The model under review builds one solid part; all positions refer to its coordinate system, in mm. Face numbers are marked on the shaded views. A direction names the side the tool comes from. Give positions to 0.01 mm unless a question says otherwise; leave off trailing zeros. Loops run counter-clockwise (first coordinate to the right, second up) from the corner with the lowest first, then second, coordinate; pieces in that order, holes last. Notation, with made-up numbers: (-28.5, 14) - (-3.5, 14) arc R20 cw to (-3.5, 26) - close; hole circle Ø4 at (57, 71). An arc over 180 degrees is marked (long way). Answer as a JSON object with one key per item and string values.
from build123d import *

# Parameters (mm, degrees)
F0_W     = 110
F0_H     = 30
F1_DEPTH = 10
F2_R     = 2
F3_DEPTH = 25
F4_W     = 10
F4_H     = 30
F5_DEPTH = 30
F6_R     = 2
F7_DEPTH = 25
F8_R     = 4.99999


# Not quite as in the source:
# - a fillet or chamfer is up to 0.001 mm smaller than in the source, because OpenCascade refuses the exact size
# - a feature names something its author has since deleted; it is built from what else it names


with BuildPart() as f1:
    # F0 (on Top) → F1 (new body)
    with BuildSketch(Plane.XY):
        with Locations((-55, 15)):
            Rectangle(F0_W, F0_H)
    extrude(amount=F1_DEPTH)

    # F2 (on face) → F3 (cut)
    with BuildSketch(Plane(origin=(0, 0, 0), x_dir=(1, 0, 0), z_dir=(0, 0, -1))):
        with Locations((-8, -8)):
            Circle(F2_R)
        with Locations((-73, -8)):
            Circle(F2_R)
        with BuildLine():
            Line((0, -30), (0, -15))
            Line((0, -15), (-65, -15))
            ThreePointArc((-65, -15), (-75.6066017178, -19.3933982822), (-80, -30))
            Line((-80, -30), (0, -30))
        make_face()
    extrude(amount=-F3_DEPTH, mode=Mode.SUBTRACT)

    # F4 (on face) → F5 (join)
    with BuildSketch(Plane.XY.offset(10)):
        with Locations((-105, 15)):
            Rectangle(F4_W, F4_H)
    extrude(amount=F5_DEPTH)

    # F6 (on face) → F7 (cut)
    with BuildSketch(Plane.YZ.offset(-100)):
        with Locations((7, 17)):
            Circle(F6_R)
        with Locations((7, 25)):
            Circle(F6_R)
        with Locations((15, 33)):
            Circle(F6_R)
        with Locations((7, 33)):
            Circle(F6_R)
        with Locations((15, 25)):
            Circle(F6_R)
        with Locations((15, 17)):
            Circle(F6_R)
        with Locations((23, 17)):
            Circle(F6_R)
        with Locations((23, 25)):
            Circle(F6_R)
        with Locations((23, 33)):
            Circle(F6_R)
    extrude(amount=-F7_DEPTH, mode=Mode.SUBTRACT)

    # F8 (radius 5 in the source; OpenCascade refuses exactly that, so slightly less here)
    f8_edges = [f1.edges().sort_by_distance(p)[0] for p in [
        (0, 15, 5),
        (0, 0, 5),
        (-80, 30, 5),
        (-105, 30, 40),
        (-105, 0, 40),
        (-100, 15, 10),
    ]]
    fillet(f8_edges, radius=F8_R)


solid = f1.part
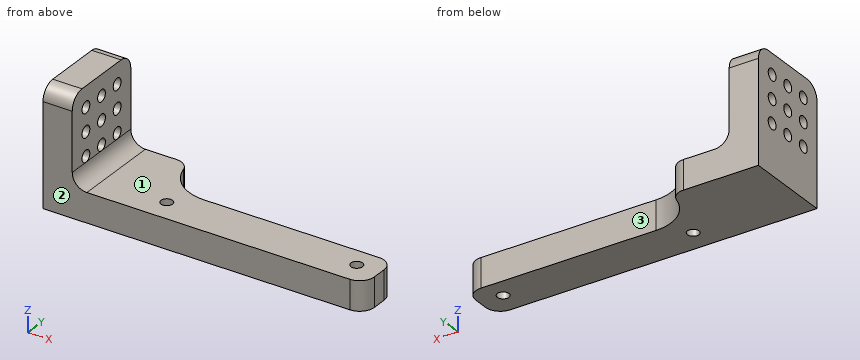
Q1. For the marked faces 1, 2 and 3, list the 3-axis set-ups (+Z, -Z, +X, -X, +Y, -Y) from which the entire face can be reached by the end or side of a thin tool; tool diameter is ignored.
Results:
{"face 1": "+Z, +X, +Y, -Y", "face 2": "+Z, -Z, +X, -X, -Y", "face 3": "+Z, -Z, +X, +Y"}
Q2. Clearance check with flat-ended pins moving along their axes: pin 1 Ø5 at (y, z) = (15, 33) entering from +X; pin 2 Ø1 at (x, y) = (-37, 6.5) entering from +Z; pin 3 Ø5 at (x, z) = (-40.5, 3.5) entering from +Y. State where each tip first meets the part, or that it passes through.
Results:
{"pin 1": "stops at x = -100", "pin 2": "stops at z = 10", "pin 3": "stops at y = 15"}
Q3. Consider section B-B, the plane x = -8. State the section outline as (y, z) points, plus the area to 3 significant figures.
Results:
{"outline": "(0, 0) - (6, 0) - (6, 10) - (0, 10) - close; (10, 0) - (15, 0) - (15, 10) - (10, 10) - close", "area": "110 mm^2"}
Q4. Consider section A-A, the plane z = 33. State the section outline as (x, y) points, plus the area to 3 significant figures.
Results:
{"outline": "(-110, 0) - (-100, 0) - (-100, 5) - (-110, 5) - close; (-110, 9) - (-100, 9) - (-100, 13) - (-110, 13) - close; (-110, 17) - (-100, 17) - (-100, 21) - (-110, 21) - close; (-110, 25) - (-100, 25) - (-100, 30) - (-110, 30) - close", "area": "180 mm^2"}
Q5. Consider section C-C, the plane y = 23. State how many separate pieces and enclosed holes the cut face has, plus the area to 3 significant figures.
Results:
{"separate pieces": "4", "enclosed holes": "0", "area": "503 mm^2"}
Q6. Consider section D-D, the plane y = 8. State the section outline as (x, z) points, plus the area to 3 significant figures.
Results:
{"outline": "(-110, 0) - (-75, 0) - (-75, 10) - (-95, 10) arc R5 cw to (-100, 15) - (-100, 15.27) - (-110, 15.27) - close; (-110, 18.73) - (-100, 18.73) - (-100, 23.27) - (-110, 23.27) - close; (-110, 26.73) - (-100, 26.73) - (-100, 31.27) - (-110, 31.27) - close; (-110, 34.73) - (-100, 34.73) - (-100, 40) - (-110, 40) - close; (-71, 0) - (-10, 0) - (-10, 10) - (-71, 10) - close; (-6, 0) - (0, 0) - (0, 10) - (-6, 10) - close", "area": "1,220 mm^2"}
Q7. To check wall thickness, follow probe 1 along Z at (x, y) = (-104.5, 15); probe 2 along X at (y, z) = (8, 6); probe 3 along Y at (x, z) = (-105, 16). State the ranges of each line that lie inside material, in increasing order. Write a range as [from, to].
Results:
{"probe 1": "z = [0, 15], [19, 23], [27, 31], [35, 40]", "probe 2": "x = [-110, -75], [-71, -10], [-6, 0]", "probe 3": "y = [0, 5.27], [8.73, 13.27], [16.73, 21.27], [24.73, 30]"}
